Print and shaded views of the part. All mm, measured from the part's lowest x, y and z. A direction names the side the tool comes from. Coordinates: 2 decimals unless noted, no trailing zeros. Write each loop counter-clockwise with the first axis right and the second up, starting at its lowest first coordinate (ties: lowest second). Pieces come first, ordered by that corner, then holes. Notation, with made-up numbers: (68, 89) -> (80, 89) arc R31 cw to (80, 117) -> close; hole circle Ø7 at (35, 1.5). An arc over 180 degrees is marked (long way). Write item = value, one per line.
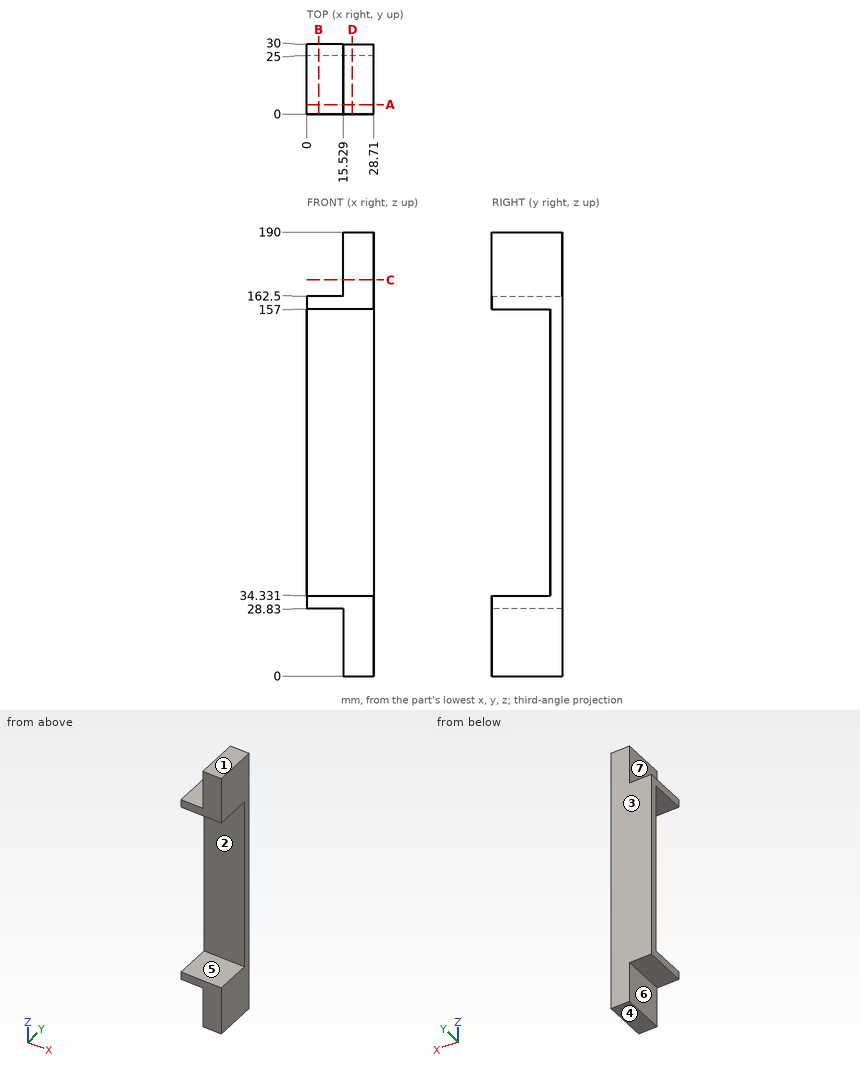
Q1. Saw through at B-B on x = 5. Give the cut face in (y, z).
Model answer:
outline = (0, 28.83) -> (30, 28.83) -> (30, 162.5) -> (0, 162.5) -> (0, 157) -> (25, 157) -> (25, 34.33) -> (0, 34.33) -> close
Q2. Probe line 1 (Z direction, x = 11.75, y = 21.75); line 2 (Z direction, x = 23.25, y = 13.75); line 3 (Y direction, x = 1.75, z = 47.5). List the from-to ranges inside material, lowest first. Write a range as from..to.
Model answer:
line_1 = 28.83..34.33, 157..162.5
line_2 = 0..34.33, 157..190
line_3 = 25..30
Q3. Pin check, flat tips, straight feed: pin 1 (4 mm diameter, centred on x = 13, y = 26, fed in from +Z); pin 2 (12.5 mm diameter, centred on x = 7.5, y = 16, fed in from -Z); pin 3 (14.5 mm diameter, centred on x = 14, z = 122, fed in from -Y). Stop position of each tip, or through.
Model answer:
pin_1 = 162.5
pin_2 = 28.83
pin_3 = 25
Q4. Saw through at D-D on x = 19.5. Give the cut face in (y, z), and give its area (3 significant figures).
Model answer:
outline = (0, 0) -> (30, 0) -> (30, 190) -> (0, 190) -> (0, 157) -> (25, 157) -> (25, 34.33) -> (0, 34.33) -> close
area = 2,630 mm²
Q5. Saw through at A-A on y = 4. Give the cut face in (x, z), and give its area (3 significant figures).
Model answer:
outline = (0, 28.83) -> (15.53, 28.83) -> (15.53, 0) -> (28.71, 0) -> (28.71, 34.33) -> (0, 34.33) -> close; (0, 157) -> (28.71, 157) -> (28.71, 190) -> (15.53, 190) -> (15.53, 162.5) -> (0, 162.5) -> close
area = 1,060 mm²
Q6. Mould opens along Z. For the marked faces 1, 2, 3 and 4 say: released by +Z, released by -Z, zero draft, split by the parting line, or undercut.
Model answer:
face_1 = released by +Z
face_2 = undercut
face_3 = zero draft
face_4 = released by -Z
Q7. Saw through at C-C on z = 169.5. Give the cut face in (x, y).
Model answer:
outline = (15.53, 0) -> (28.71, 0) -> (28.71, 30) -> (15.53, 30) -> close
Q8. Which spindle directions (+Z, -Z, +X, -X, +Y, -Y) get a long thin tool onto all of the face, cutting with end or side? Do the marked faces 5, 6 and 7. Say none if no direction does.
Model answer:
face_5 = +X, -X, -Y
face_6 = -Z, -X, +Y, -Y
face_7 = +Z, -X, +Y, -Y
